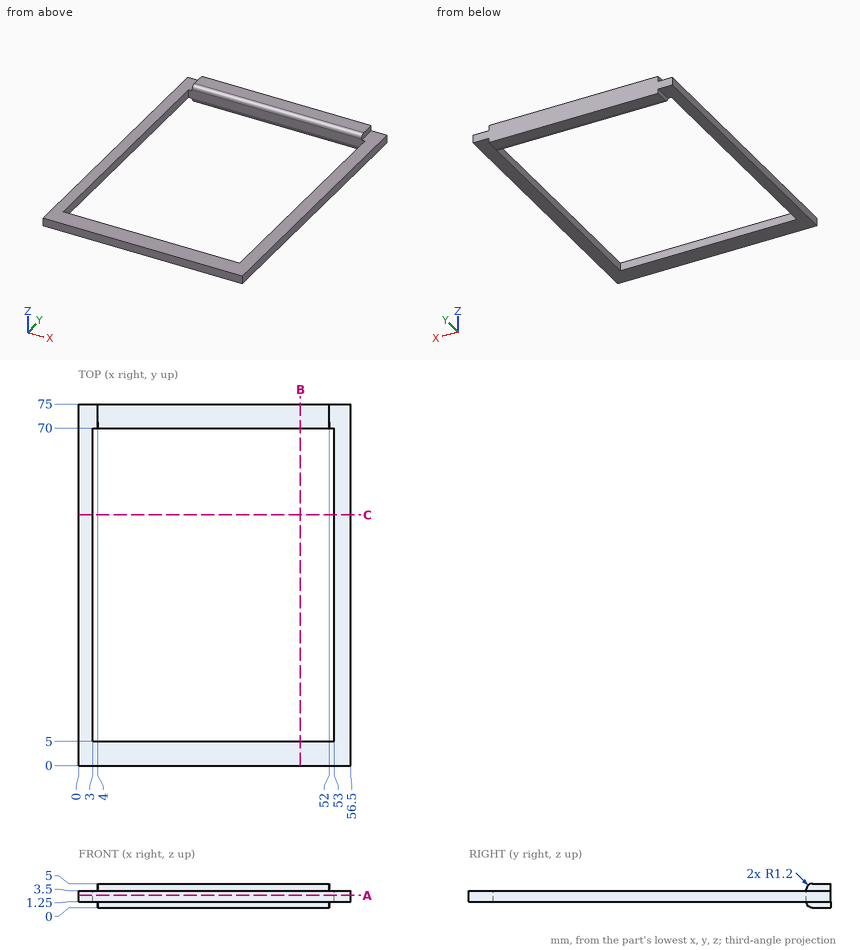
The drawing under review shows one solid part. Ordinate dimensions are in mm from its lowest x, y, z. Coordinates: 2 decimals unless noted, no trailing zeros. Order: outer loops, then holes, each group sorted by start corner. A loop starts at its lowest first (then second) coordinate and runs counter-clockwise, first axis right, second up. Notation, with made-up numbers: (83.25, 47.5) -> (90.25, 47.5) arc R8 ccw to (90.25, 58.5) -> close; hole circle Ø8 at (33.5, -20.5). An arc over 180 degrees is marked (long way). Use CSV: the item, a comma, the result in double quotes. Start each with the question number.
Item 1: We need section B-B, the plane x = 46. Give the boundary of the cut face in (y, z).
Item 2: Insertion check: pin 1 (0.6 mm diameter, centred on y = 72.5, z = 1, fed in from -X); pin 2 (1.7 mm diameter, centred on y = 73.5, z = 4.5, fed in from +X). Each pin has a flat end and moves straight along its axis. Give the tip position at first contact, or say it passes through.
Item 3: We need section A-A, the plane z = 2.55. Give the boundary of the cut face in (x, y).
Item 4: Wall thickness on probe 1 along X at (y, z) = (39, 2.7); probe 2 along Y at (x, z) = (17, 1.6); probe 3 along Y at (x, z) = (5, 0.35): over which ranges is each line inside the solid? List them lowest first.
Item 5: We need section C-C, the plane y = 52. Give the boundary of the cut face in (x, z).
Derived:
1,outline,"(0, 1.25) -> (5, 1.25) -> (5, 3.5) -> (0, 3.5) -> close; (70, 1.2) arc R1.2 ccw to (71.2, 0) -> (75, 0) -> (75, 5) -> (71.2, 5) arc R1.2 ccw to (70, 3.8) -> close"
2,pin 1,"stops at x = 0"
2,pin 2,"stops at x = 52"
3,outline,"(0, 0) -> (56.5, 0) -> (56.5, 75) -> (0, 75) -> close; hole (3, 5) -> (53, 5) -> (53, 70) -> (3, 70) -> close"
4,probe 1,"x = 0 to 3, 53 to 56.5"
4,probe 2,"y = 0 to 5, 70 to 75"
4,probe 3,"y = 70.35 to 75"
5,outline,"(0, 1.25) -> (3, 1.25) -> (3, 3.5) -> (0, 3.5) -> close; (53, 1.25) -> (56.5, 1.25) -> (56.5, 3.5) -> (53, 3.5) -> close"
